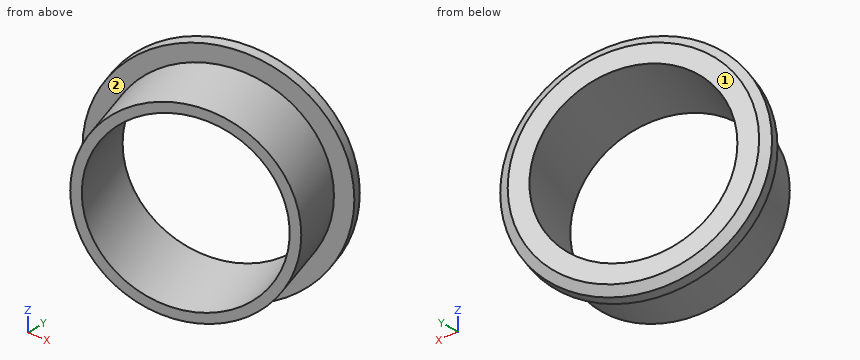
```python
from build123d import *


with BuildPart() as part:
    # Sk_Cono → Cono (revolve)
    with BuildSketch(Plane.XY, mode=Mode.PRIVATE) as cono_sk:
        Polygon((385.500399814, 520.056357213), (387.121714083, 520.567571493), (383.513142692, 532.012142805), (386.37428552, 532.914285653), (385.772856954, 534.821714205), (384.041571258, 535.324357057), (380.989685575, 534.362071352), align=None)
    revolve(cono_sk.sketch.rotate(Axis((364.894285739, 534.529714208, 0), (0.3007142826457708, -0.9537142759825081, 0)), 180), axis=Axis((364.894285739, 534.529714208, 0), (0.3007142826457708, -0.9537142759825081, 0)))


solid = part.part
```
The listing builds one solid part. Answer for the finished solid, in the listing's coordinates (mm). Face numbers are marked on the shaded views. Give positions to 0.01 mm unless a question says otherwise; leave off trailing zeros. Answer as a JSON object with one key per item and string values. Group by question number.
Item 1: Flat-ended cylindrical pins translate along their axes: pin 1 (4 mm diameter, centred on y = 518.5, z = -16, fed in from -X); pin 2 (6 mm diameter, centred on x = 365, y = 523.5, fed in from +Z); pin 3 (3 mm diameter, centred on x = 377.5, y = 524.5, fed in from +Z). Find the tip coordinate at first contact, or state that the pin passes through.
Item 2: Determine the mould class of the marked faces 1 and 2 for opening direction Y: pulls with the +Y half, pulls with the -Y half, needs draft (parallel to the pull), parting line crosses it, or undercut.
Item 3: Consider L1, parallel to Z at x = 372, y = 530.5; L2, parallel to Z at x = 366, y = 525; L3, parallel to X at y = 523.75, z = -13. Determine where each line is inside the solid, lowest interval first. Write a range as from..to.
Result set:
{
 "1": {"pin 1": "x = 359.77", "pin 2": "z = 19.93", "pin 3": "z = 15.25"},
 "2": {"face 1": "pulls with the +Y half", "face 2": "undercut"},
 "3": {"L1": "-19.18..-14.25, 14.25..19.18", "L2": "-16.9..-15.19, 15.19..16.9", "L3": "352.36..359.83, 376.75..379.78"}
}
